Could you check a few things on this model? Use its own coordinates, in mm. Coordinates: 2 decimals unless noted, no trailing zeros. Loops run counter-clockwise (first coordinate to the right, second up) from the corner with the lowest first, then second, coordinate; pieces in that order, holes last. Notation, with made-up numbers: (53.25, 87.5) - (68.25, 87.5) arc R26 cw to (68.25, 108.5) - close; hole circle Ø5 at (29.5, 25.5). An arc over 180 degrees is marked (long way). Use CSV: the item, a comma, the result in double quotes.
from build123d import *

# Parameters (mm, degrees)
SKETCH_1_W      = 228
SKETCH_1_H      = 84
SKETCH_1_R      = 2.6
SKETCH_1_R_2    = 2.15
EXTRUDE_1_DEPTH = 1


with BuildPart() as part:
    # Эскиз1 → Вытянуть1 (new body)
    with BuildSketch(Plane.XY):
        Rectangle(SKETCH_1_W, SKETCH_1_H)
        with Locations((-42.5, 0)):
            Circle(SKETCH_1_R, mode=Mode.SUBTRACT)
        with Locations((42.5, 0)):
            Circle(SKETCH_1_R, mode=Mode.SUBTRACT)
        with Locations((107, 32)):
            Circle(SKETCH_1_R_2, mode=Mode.SUBTRACT)
        with Locations(Location((-107, 32, 0), (0, 0, 180))):
            Circle(SKETCH_1_R_2, mode=Mode.SUBTRACT)
        with Locations((-107, -32)):
            Circle(SKETCH_1_R_2, mode=Mode.SUBTRACT)
        with Locations(Location((107, -32, 0), (0, 0, 180))):
            Circle(SKETCH_1_R_2, mode=Mode.SUBTRACT)
    extrude(amount=EXTRUDE_1_DEPTH)


solid = part.part
(1) Please list where these lines run through material, in increasing order: line 1 (Y direction, x = -107, z = 0.3); line 2 (Y direction, x = 42.5, z = 0.85); line 3 (Y direction, x = -43.5, z = 0.55).
Computed:
line 1,"y = -42 to -34.15, -29.85 to 29.85, 34.15 to 42"
line 2,"y = -42 to -2.6, 2.6 to 42"
line 3,"y = -42 to -2.4, 2.4 to 42"
(2) Suppose I cut it at A-A (y = 32). Write out the boundary of the cut face in (x, z), plus the area to 3 significant figures.
Computed:
outline,"(-114, 0) - (-109.15, 0) - (-109.15, 1) - (-114, 1) - close; (-104.85, 0) - (104.85, 0) - (104.85, 1) - (-104.85, 1) - close; (109.15, 0) - (114, 0) - (114, 1) - (109.15, 1) - close"
area,"219 mm²"
(3) Suppose I cut it at C-C (x = -42.5). Write out the boundary of the cut face in (y, z).
Computed:
outline,"(-42, 0) - (-2.6, 0) - (-2.6, 1) - (-42, 1) - close; (2.6, 0) - (42, 0) - (42, 1) - (2.6, 1) - close"
(4) Suppose I cut it at B-B (x = 107). Write out the boundary of the cut face in (y, z), plus the area to 3 significant figures.
Computed:
outline,"(-42, 0) - (-34.15, 0) - (-34.15, 1) - (-42, 1) - close; (-29.85, 0) - (29.85, 0) - (29.85, 1) - (-29.85, 1) - close; (34.15, 0) - (42, 0) - (42, 1) - (34.15, 1) - close"
area,"75.4 mm²"
(5) Will this pin go through, and if not, where does the flat tip stop? pin 1 (3.5 mm diameter, centred on x = -107, y = 32, fed in from -Z).
Computed:
pin 1,"passes through"
(6) Thinking about a two-plate mould opening in X: for faces 1 (the face through (105.415, 33.453, 0.493)), 2 (the face through (-108.585, -30.547, 0.493)), 3 (the face through (-2, 1, 1)), which applies, +X half, -X half, draft (parallel to the pull), parting line (faces both ways), or undercut?
Computed:
face 1,"undercut"
face 2,"undercut"
face 3,"draft"
